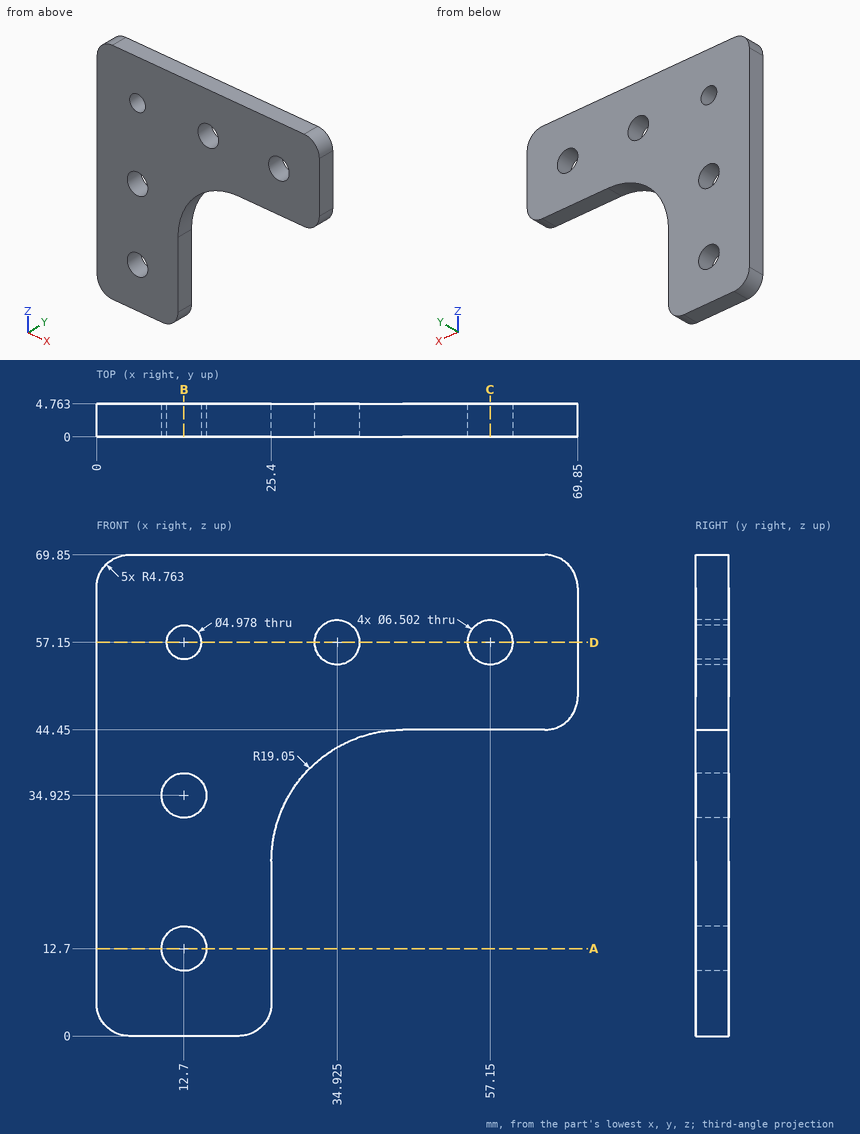
Here's the drawing with two shaded views (mm, measured from the low corner). I have some questions. Round coordinates to 2 decimals unless told otherwise and drop trailing zeros. Loops run counter-clockwise (first coordinate to the right, second up) from the corner with the lowest first, then second, coordinate; pieces in that order, holes last.
Item 1: Will these pins go through, and if not, where does the flat tip stop? pin 1 Ø5.5 at (x, z) = (12.7, 57.15) entering from +Y; pin 2 Ø2 at (x, y) = (57.5, 1.5) entering from -Z.
Item 2: Suppose I cut it at B-B, the plane x = 12.7. Write out the boundary of the cut face in (y, z).
Item 3: Suppose I cut it at A-A, the plane z = 12.7. Write out the boundary of the cut face in (x, y).
Item 4: Suppose I cut it at D-D, the plane z = 57.15. Write out the boundary of the cut face in (x, y).
Item 5: Suppose I cut it at C-C, the plane x = 57.15. Write out the boundary of the cut face in (y, z).
Item 6: Please list where these lines run through material, in increasing order: L1, parallel to Z at x = 12.7, y = 2.8; L2, parallel to Z at x = 57.15, y = 3.75; L3, parallel to Z at x = 63, y = 2.9.
Reported:
1. pin 1: stops at y = 4.76
1. pin 2: stops at z = 44.45
2. outline: (0, 0) - (4.76, 0) - (4.76, 9.45) - (0, 9.45) - close; (0, 15.95) - (4.76, 15.95) - (4.76, 31.67) - (0, 31.67) - close; (0, 38.18) - (4.76, 38.18) - (4.76, 54.66) - (0, 54.66) - close; (0, 59.64) - (4.76, 59.64) - (4.76, 69.85) - (0, 69.85) - close
3. outline: (0, 0) - (9.45, 0) - (9.45, 4.76) - (0, 4.76) - close; (15.95, 0) - (25.4, 0) - (25.4, 4.76) - (15.95, 4.76) - close
4. outline: (0, 0) - (10.21, 0) - (10.21, 4.76) - (0, 4.76) - close; (15.19, 0) - (31.67, 0) - (31.67, 4.76) - (15.19, 4.76) - close; (38.18, 0) - (53.9, 0) - (53.9, 4.76) - (38.18, 4.76) - close; (60.4, 0) - (69.85, 0) - (69.85, 4.76) - (60.4, 4.76) - close
5. outline: (0, 44.45) - (4.76, 44.45) - (4.76, 53.9) - (0, 53.9) - close; (0, 60.4) - (4.76, 60.4) - (4.76, 69.85) - (0, 69.85) - close
6. L1: z = 0 to 9.45, 15.95 to 31.67, 38.18 to 54.66, 59.64 to 69.85
6. L2: z = 44.45 to 53.9, 60.4 to 69.85
6. L3: z = 44.45 to 69.85
